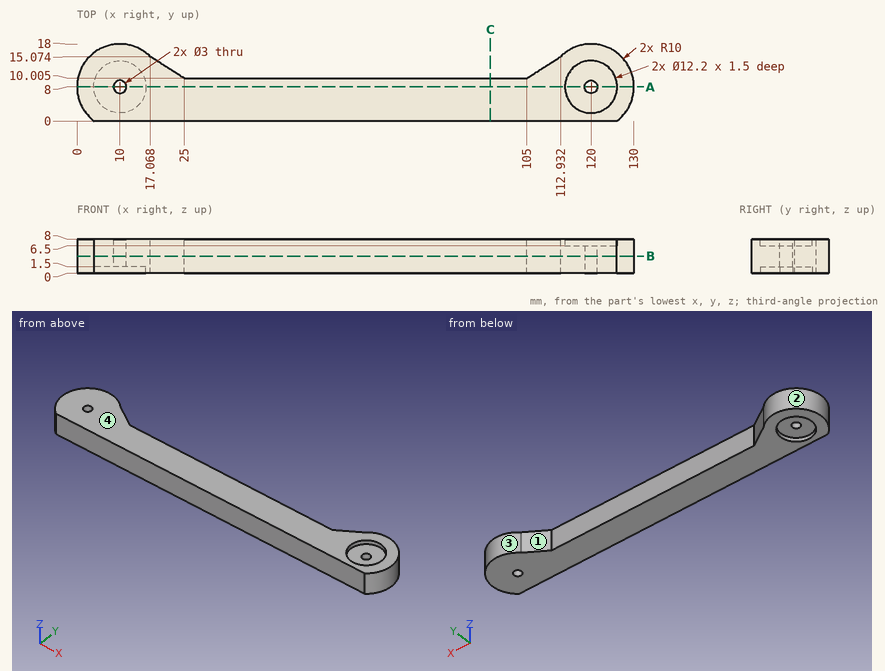
Geometry check sheet. Reference: drawing and pictorial views, mm from the part's lowest x, y, z. A direction names the side the tool comes from. Give positions to 0.01 mm unless a question says otherwise; leave off trailing zeros. Write each loop counter-clockwise with the first axis right and the second up, starting at its lowest first coordinate (ties: lowest second). Pieces come first, ordered by that corner, then holes. Notation, with made-up numbers: (57, -36.5) -> (93, -36.5) arc R23 cw to (93, -13.5) -> close; hole circle Ø2 at (66.25, 29.5). An arc over 180 degrees is marked (long way). One line per item, written item: value. Start each with the question number.
Item 1: Section check A-A on y = 8. Record the cut outline in (x, z).
Item 2: Section check B-B on z = 4. Record the cut outline in (x, y) (1 decimal).
Item 3: Gauge pin test, flat ends, axial feed: pin 1 (10 mm diameter, centred on x = 8.5, y = 6.5, fed in from -Z); pin 2 (4 mm diameter, centred on x = 46.5, z = 4.5, fed in from +Y) (3 decimals); pin 3 (4 mm diameter, centred on y = 5, z = 1.5, fed in from +X). Record the tip position at first contact, or that the pin passes through.
Item 4: Material ranges on probe 1 along X at (y, z) = (8, 6); probe 2 along X at (y, z) = (8, 0.6); probe 3 along Y at (x, z) = (81.5, 4.5) (1 decimal), recorded low to high. Write a range as from..to.
Item 5: Draft check along X on the marked faces 3 and 4. Enter one of: +X half, -X half, draft (parallel to the pull), parting line (faces both ways), or undercut.
Item 6: Tool access check on the marked faces 1 and 2. Record the directions out of +Z, -Z, +X, -X, +Y, -Y that give a thin tool (end or side, any length) a straight path to the whole face; none if there is none.
Item 7: Section check C-C on x = 96.5. Record the cut outline in (y, z) (1 decimal).
Results list:
1. outline: (0, 0) -> (3.9, 0) -> (3.9, 1.5) -> (8.5, 1.5) -> (8.5, 8) -> (0, 8) -> close; (11.5, 1.5) -> (16.1, 1.5) -> (16.1, 0) -> (118.5, 0) -> (118.5, 6.5) -> (113.9, 6.5) -> (113.9, 8) -> (11.5, 8) -> close; (121.5, 0) -> (130, 0) -> (130, 8) -> (126.1, 8) -> (126.1, 6.5) -> (121.5, 6.5) -> close
2. outline: (4, 0) -> (126, 0) arc R10 ccw (long way) to (112.9, 15.1) -> (105, 10) -> (25, 10) -> (17.1, 15.1) arc R10 ccw (long way) to start; hole circle Ø3 at (10, 8); hole circle Ø3 at (120, 8)
3. pin 1: z = 0
3. pin 2: y = 10.005
3. pin 3: x = 129.95
4. probe 1: 0..8.5, 11.5..118.5, 121.5..130
4. probe 2: 0..3.9, 16.1..118.5, 121.5..130
4. probe 3: 0..10
5. face 3: undercut
5. face 4: draft
6. face 1: +Z, -Z, +Y
6. face 2: +Z, -Z
7. outline: (0, 0) -> (10, 0) -> (10, 8) -> (0, 8) -> close
